Source: CAD feature listing. Evaluate the final solid. Frame: model axes, mm. Face numbers are marked on the shaded views. A direction names the side the tool comes from. Give positions to 0.01 mm unless a question says otherwise; leave off trailing zeros. Loops run counter-clockwise (first coordinate to the right, second up) from the corner with the lowest first, then second, coordinate; pieces in that order, holes last. Notation, with made-up numbers: (59.5, -24) -> (92.5, -24) arc R17 cw to (92.5, -19) -> close; hole circle Ø8 at (70, -37.5). An arc over 180 degrees is marked (long way). Return JSON: item names as keys, results as strings. Group by question number.
```python
from build123d import *

# Parameters (mm, degrees)
BOSS_EXTRUDE1_DEPTH = 5
SKETCH2_W           = 3.3
SKETCH2_H           = 6
CUT_EXTRUDE2_DEPTH  = 6.5
SKETCH3_R           = 2.15
CUT_EXTRUDE4_DEPTH  = 24
FILLET1_R           = 0.5
FILLET2_R           = 3
BOSS_EXTRUDE2_DEPTH = 7
FILLET3_R           = 3


with BuildPart() as part:
    # Sketch1 → Boss-Extrude1 (new, symmetric)
    with BuildSketch(Plane.XY):
        with BuildLine():
            Line((40, -13), (34.35, -13))
            Line((34.35, -13), (34.35, 3))
            ThreePointArc((34.35, 3), (26.182605601, 5.085665361), (32.35, -0.660601044))
            Line((32.35, -0.660601044), (32.35, -13))
            Line((32.35, -13), (7.5, -13))
            Line((7.5, -13), (7.5, -6))
            Line((7.5, -6), (5.1, -6))
            Line((5.1, -6), (5.1, -13))
            Line((5.1, -13), (-5.1, -13))
            Line((-5.1, -13), (-5.1, -6))
            Line((-5.1, -6), (-7.5, -6))
            Line((-7.5, -6), (-7.5, -13))
            Line((-7.5, -13), (-32.35, -13))
            Line((-32.35, -13), (-32.35, -0.660601044))
            ThreePointArc((-32.35, -0.660601044), (-26.182605601, 5.085665361), (-34.35, 3))
            Line((-34.35, 3), (-34.35, -13))
            Line((-34.35, -13), (-40, -13))
            Line((-40, -13), (-40, 13))
            Line((-40, 13), (40, 13))
            Line((40, 13), (40, -13))
        make_face()
    extrude(amount=BOSS_EXTRUDE1_DEPTH, both=True)

    # Sketch2 → Cut-Extrude2 (cut)
    with BuildSketch(Plane.XY.offset(5)):
        with Locations((-24, -10)):
            Rectangle(SKETCH2_W, SKETCH2_H)
        with Locations((24, -10)):
            Rectangle(SKETCH2_W, SKETCH2_H)
    extrude(amount=-CUT_EXTRUDE2_DEPTH, mode=Mode.SUBTRACT)

    # Sketch3 → Cut-Extrude4 (cut)
    with BuildSketch(Plane.ZY.offset(40)):
        with Locations(Location((2, -10, 0), (0, 0, 180))):
            Circle(SKETCH3_R)
    cut_extrude4 = extrude(amount=-CUT_EXTRUDE4_DEPTH, mode=Mode.SUBTRACT)

    # Mirror1: Cut-Extrude4 across plane
    add(cut_extrude4.mirror(Plane(origin=(0, 0, 0), x_dir=(0, 0, 1), z_dir=(1, 0, 0))), mode=Mode.SUBTRACT)

    # Fillet1
    fillet1_edges = [part.edges().sort_by_distance(p)[0] for p in [
        (5.1, -9.5, -5),
        (-5.1, -9.5, -5),
    ]]
    fillet(fillet1_edges, radius=FILLET1_R)

    # Fillet2
    fillet2_edges = [part.edges().sort_by_distance(p)[0] for p in [
        (-40, 13, 0),
        (40, 13, 0),
    ]]
    fillet(fillet2_edges, radius=FILLET2_R)

    # Sketch4 → Boss-Extrude2 (add)
    with BuildSketch(Plane.XZ.offset(13)):
        with BuildLine():
            Line((-5.1, 5), (5.1, 5))
            ThreePointArc((5.1, 5), (0, 7.142128534), (-5.1, 5))
        make_face()
    extrude(amount=-BOSS_EXTRUDE2_DEPTH)

    # Fillet3
    # the kernel refuses this fillet: 3 mm, written as the material it adds along each edge
    with BuildSketch(Plane(origin=(-12.6, -6, 5), x_dir=(0, 1, 0), z_dir=(1, 0, 0))) as fillet3_piece_1_section:
        with BuildLine():
            CenterArc((FILLET3_R, FILLET3_R), FILLET3_R, 180, 90)
            Line((0, FILLET3_R), (0, 0))
            Line((0, 0), (FILLET3_R, 0))
        make_face()
    fillet3_piece_1 = extrude(amount=25.2, mode=Mode.PRIVATE)
    fillet3_piece_1 = fillet3_piece_1 & Plane(origin=(0, -5.25920744, 0), x_dir=(0.7140728391445785, 0, 0.7000714109260576), z_dir=(0, -1, 0)) * Cylinder(7.142128534, 63, mode=Mode.PRIVATE)
    add(fillet3_piece_1)


solid = part.part
```
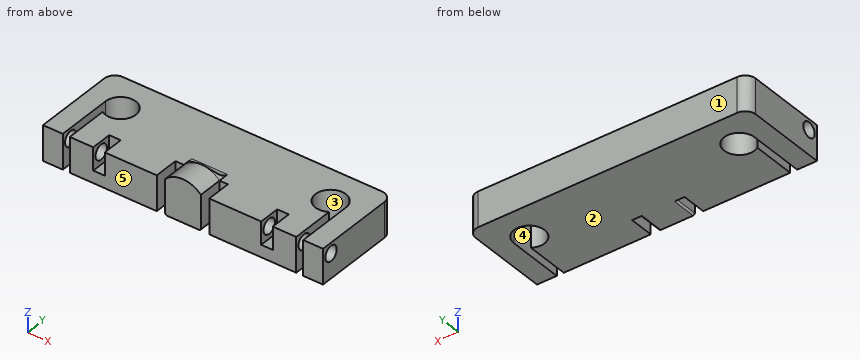
1) Cut plane D-D on x = -3. Return loops of the section in (y, z).
2) Cut plane A-A on x = -30. Return loops of the section in (y, z).
3) Cut plane C-C on z = -2.5. Return loops of the section in (x, y).
4) Mould query, pull axis Y, two halves, no side actions, for the marked faces 1, 2 and 3. Classes: released by +Y, released by -Y, zero draft, split by the parting line, or undercut.
5) Contact query for flat-ended pins moving along their axis: P1, Ø4, axis at y = -10, z = 2, coming from the +X side; P2, Ø6, axis at x = -5, y = 3.5, coming from the +Z side. Output: stop coordinate, or through.
6) Reachability of the marked faces 4 and 5 from +Z, -Z, +X, -X, +Y, -Y: full face, straight path, thin tool, end or side. Return the list, or none.
7) Material intervals for line 1 (X direction, y = -12, z = -3.5); line 2 (X direction, y = -12, z = 2.5); line 3 (X direction, y = -5, z = -1.5), sorted ascending.
8) Cut plane B-B on y = 1.25. Return loops of the section in (x, z).
Calculated:
{
 "1": {"outline": "(-13, -5) -> (13, -5) -> (13, 5) -> (-3, 5) arc R3 cw to (-5.59, 6.48) -> (-13, 6.48) -> close"},
 "2": {"outline": "(-13, -5) -> (-1.35, -5) -> (-1.35, 5) -> (-13, 5) -> close; (7.35, -5) -> (13, -5) -> (13, 5) -> (7.35, 5) -> close; hole circle Ø4.3 at (-10, 2)"},
 "3": {"outline": "(-40, -13) -> (-34.35, -13) -> (-34.35, 3) arc R4.35 cw (long way) to (-32.35, -0.66) -> (-32.35, -13) -> (-7.5, -13) -> (-7.5, -6) -> (-5.1, -6) -> (-5.1, -13) -> (5.1, -13) -> (5.1, -6) -> (7.5, -6) -> (7.5, -13) -> (32.35, -13) -> (32.35, -0.66) arc R4.35 cw (long way) to (34.35, 3) -> (34.35, -13) -> (40, -13) -> (40, 10) arc R3 ccw to (37, 13) -> (-37, 13) arc R3 ccw to (-40, 10) -> close"},
 "4": {"face 1": "released by +Y", "face 2": "zero draft", "face 3": "undercut"},
 "5": {"P1": "x = 16", "P2": "z = 5"},
 "6": {"face 4": "+Z, -Z, -Y", "face 5": "+Z, -Z, +X, -X, -Y"},
 "7": {"line 1": "-40 to -34.35, -32.35 to -7.5, -5.1 to 5.1, 7.5 to 32.35, 34.35 to 40", "line 2": "-16 to -7.5, -5.1 to 5.1, 7.5 to 16", "line 3": "-40 to -34.35, -32.35 to 32.35, 34.35 to 40"},
 "8": {"outline": "(-40, -5) -> (-34.35, -5) -> (-34.35, 5) -> (-40, 5) -> close; (-26.02, -5) -> (26.02, -5) -> (26.02, 5) -> (-26.02, 5) -> close; (34.35, -5) -> (40, -5) -> (40, 5) -> (34.35, 5) -> close"}
}
